Verification items for this drawing (mm, ordinates from the low corner). A direction names the side the tool comes from. Round coordinates to 2 decimals unless told otherwise and drop trailing zeros. Order: outer loops, then holes, each group sorted by start corner. A loop starts at its lowest first (then second) coordinate and runs counter-clockwise, first axis right, second up. Notation, with made-up numbers: (62.5, 0.5) - (91.5, 0.5) arc R12 cw to (91.5, 6.5) - close; hole circle Ø1 at (-32.75, -11.5). An arc over 180 degrees is marked (long way). Use a Markdown table: item, result. Add a question column.
(1) Section check A-A on y = 73. Record the boundary of the cut face in (x, z) (1 decimal).
(2) Section check C-C on x = 36.5. Record the boundary of the cut face in (y, z) (1 decimal), then the cut area to 3 significant figures.
(3) Gauge pin test, flat ends, axial feed: P1, Ø12.5, axis at y = 85, z = 16.5, coming from the -X side; P2, Ø10, axis at x = 20, z = 12, coming from the +Y side; P3, Ø4, axis at x = 17.5, z = 15.5, coming from the -Y side. Record the tip position at first contact, or that the pin passes through.
(4) Thickness scan on line 1 along Y through (x, z) = (2.4, 12.7); line 2 along X through (y, z) = (24, 31) (1 decimal); line 3 along Y through (x, z) = (20, 42). Record the ranges inside material, lowest first. Write a range as [from, to].
(5) Access from +Z, -Z, +X, -X, +Y, -Y to the whole of each face (thin tool, end or side, straight path). Record for the marked faces 1, 2 and 3.
(6) Section check B-B on x = 20. Record the boundary of the cut face in (y, z), then the cut area to 3 significant figures.
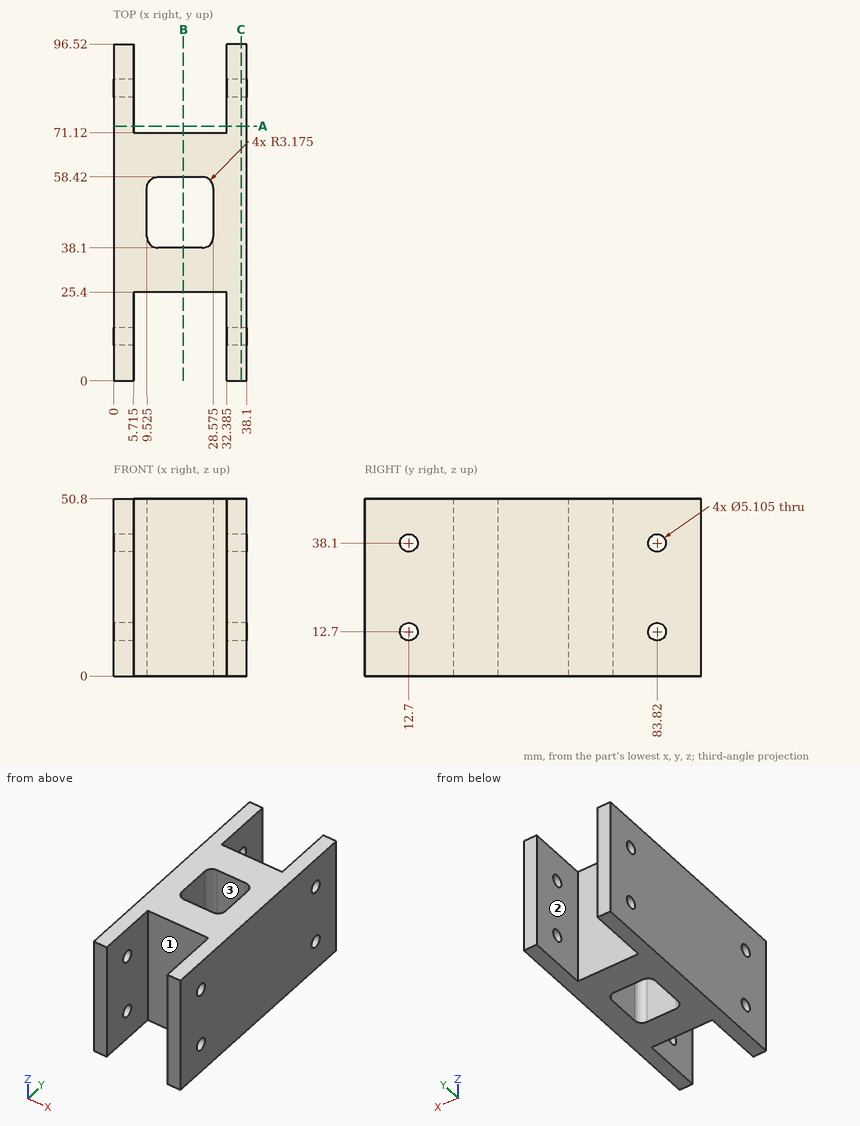
Check sheet entries:
| question | item | result |
|---|---|---|
| 1 | outline | (0, 0) - (5.7, 0) - (5.7, 50.8) - (0, 50.8) - close; (32.4, 0) - (38.1, 0) - (38.1, 50.8) - (32.4, 50.8) - close |
| 2 | outline | (0, 0) - (96.5, 0) - (96.5, 50.8) - (0, 50.8) - close; hole circle Ø5.1 at (12.7, 12.7); hole circle Ø5.1 at (12.7, 38.1); hole circle Ø5.1 at (83.8, 12.7); hole circle Ø5.1 at (83.8, 38.1) |
| 2 | area | 4,820 mm2 |
| 3 | P1 | stops at x = 0 |
| 3 | P2 | stops at y = 71.12 |
| 3 | P3 | stops at y = 25.4 |
| 4 | line 1 | y = [0, 10.15], [15.25, 81.27], [86.37, 96.52] |
| 4 | line 2 | x = [0, 5.7], [32.4, 38.1] |
| 4 | line 3 | y = [25.4, 38.1], [58.42, 71.12] |
| 5 | face 1 | +Z, -Z, -Y |
| 5 | face 2 | +Z, -Z, +Y |
| 5 | face 3 | +Z, -Z |
| 6 | outline | (25.4, 0) - (38.1, 0) - (38.1, 50.8) - (25.4, 50.8) - close; (58.42, 0) - (71.12, 0) - (71.12, 50.8) - (58.42, 50.8) - close |
| 6 | area | 1,290 mm2 |
